Here's how the part is built. I have some questions about the finished solid (model axes, mm). A direction names the side the tool comes from. Round coordinates to 2 decimals unless told otherwise and drop trailing zeros. Loops run counter-clockwise (first coordinate to the right, second up) from the corner with the lowest first, then second, coordinate; pieces in that order, holes last. Notation, with made-up numbers: (56.25, 27) -> (110.25, 27) arc R31 ccw to (110.25, 55) -> close; hole circle Ø3 at (-34, 82.5). An arc over 180 degrees is marked (long way). Use one line per item in the form item = value. Start each with the question number.
Item 1: For faces 1 (the face through (42, 2, 68)), 2 (the face through (-93, 2, -10)), 3 (the face through (-80, 2, 1)), which set-ups out of +Z, -Z, +X, -X, +Y, -Y let a thin tool reach every point of the face, with its end or its side?
Item 2: I'm going to push flat-ended pins straight in: pin 1 Ø2.5 at (x, y) = (-44.5, 3) entering from +Z; pin 2 Ø2.5 at (x, y) = (72.5, 3) entering from +Z; pin 3 Ø1.9 at (x, z) = (-78, -48) entering from +Y; pin 4 Ø2.5 at (y, z) = (3, 36) entering from -X. Where does each tip first touch, or does it pass through?
Item 3: If we section it at B-B (z = 15): Write out the boundary of the cut face in (x, y).
Item 4: If I drill on L1, parallel to Z at x = -78, y = 2.4; L2, parallel to Z at x = 44.9, y = 4.05; L3, parallel to X at y = 4.6, z = -71.5, over which ranges is the centre line in solid material (lowest first)? Write a range as [from, to].
Item 5: Thinking about a two-plate mould opening in Z: for faces 4 (the face through (0, 2, 75)), 5 (the face through (100, 2, -48)), 6 (the face through (68, 2, -68)), which applies, released by +Z, released by -Z, zero draft, split by the parting line, or undercut?
Item 6: If we section it at A-A (x = 71): Write out the boundary of the cut face in (y, z), then the cut area to 3 significant figures.
Item 7: If we section it at C-C (y = 3.7): State how many separate pieces and enclosed holes the cut face has, then the cut area to 3 significant figures.
```python
from build123d import *

# Parameters (mm, degrees)
SKETCH1_R           = 1.55
SKETCH1_W           = 20
SKETCH1_H           = 15
SKETCH1_W_2         = 5
SKETCH1_H_2         = 25
BOSS_EXTRUDE2_DEPTH = 5


with BuildPart() as part:
    # Sketch1 → Boss-Extrude2 (new body)
    with BuildSketch(Plane(origin=(0, 0, 0), x_dir=(1, 0, 0), z_dir=(0, 1, 0))):
        Polygon((-25, -75), (25, -75), (25, -68), (60, -68), (60, -1), (100, -1), (100, 0), (100, 98), (-100, 98), (-100, 0), (-100, -1), (-60, -1), (-60, -68), (-25, -68), align=None)
        with Locations((-78, 48)):
            Circle(SKETCH1_R, mode=Mode.SUBTRACT)
        with Locations((78, 48)):
            Circle(SKETCH1_R, mode=Mode.SUBTRACT)
        with Locations((-40, 48)):
            Circle(SKETCH1_R, mode=Mode.SUBTRACT)
        with Locations((40, 48)):
            Circle(SKETCH1_R, mode=Mode.SUBTRACT)
        with Locations((-44.9, 26.9)):
            Circle(SKETCH1_R, mode=Mode.SUBTRACT)
        with Locations((44.9, 26.9)):
            Circle(SKETCH1_R, mode=Mode.SUBTRACT)
        with Locations((-44.9, -62.9)):
            Circle(SKETCH1_R, mode=Mode.SUBTRACT)
        with Locations((-44.9, -20.1)):
            Circle(SKETCH1_R, mode=Mode.SUBTRACT)
        with Locations((-54.9, -62.9)):
            Circle(SKETCH1_R, mode=Mode.SUBTRACT)
        with Locations((-54.9, -20.1)):
            Circle(SKETCH1_R, mode=Mode.SUBTRACT)
        with Locations((44.9, -62.9)):
            Circle(SKETCH1_R, mode=Mode.SUBTRACT)
        with Locations((54.9, -62.9)):
            Circle(SKETCH1_R, mode=Mode.SUBTRACT)
        with Locations((44.9, -20.1)):
            Circle(SKETCH1_R, mode=Mode.SUBTRACT)
        with Locations((54.9, -20.1)):
            Circle(SKETCH1_R, mode=Mode.SUBTRACT)
        with Locations((-55, 48)):
            Circle(SKETCH1_R, mode=Mode.SUBTRACT)
        with Locations((55, 48)):
            Circle(SKETCH1_R, mode=Mode.SUBTRACT)
        with Locations((-26.7, 10.2)):
            Circle(SKETCH1_R, mode=Mode.SUBTRACT)
        with Locations((26.7, 10.2)):
            Circle(SKETCH1_R, mode=Mode.SUBTRACT)
        with Locations((-40.5, 3.605469995)):
            Circle(SKETCH1_R, mode=Mode.SUBTRACT)
        with Locations((40.5, 3.605469995)):
            Circle(SKETCH1_R, mode=Mode.SUBTRACT)
        with Locations((-23, 53.5)):
            Circle(SKETCH1_R, mode=Mode.SUBTRACT)
        with Locations((23, 53.5)):
            Circle(SKETCH1_R, mode=Mode.SUBTRACT)
        with Locations((-55, 42)):
            Circle(SKETCH1_R, mode=Mode.SUBTRACT)
        with Locations((-55, 36)):
            Circle(SKETCH1_R, mode=Mode.SUBTRACT)
        with Locations((55, 36)):
            Circle(SKETCH1_R, mode=Mode.SUBTRACT)
        with Locations((55, 42)):
            Circle(SKETCH1_R, mode=Mode.SUBTRACT)
        with Locations((-78, 68.5)):
            Rectangle(SKETCH1_W, SKETCH1_H, mode=Mode.SUBTRACT)
        with Locations((78, 68.5)):
            Rectangle(SKETCH1_W, SKETCH1_H, mode=Mode.SUBTRACT)
        with Locations((-92.5, 22.5)):
            Rectangle(SKETCH1_W_2, SKETCH1_H_2, mode=Mode.SUBTRACT)
        with Locations((92.5, 22.5)):
            Rectangle(SKETCH1_W_2, SKETCH1_H_2, mode=Mode.SUBTRACT)
    extrude(amount=BOSS_EXTRUDE2_DEPTH)


solid = part.part
```
Values found:
q1.face_1 = +Z, +X, +Y, -Y
q1.face_2 = +Y, -Y
q1.face_3 = +Z, -X, +Y, -Y
q2.pin_1 = 68
q2.pin_2 = 1
q2.pin_3 = through
q2.pin_4 = -60
q3.outline = (-60, 0) -> (60, 0) -> (60, 5) -> (-60, 5) -> close
q4.L1 = [-98, -76], [-61, -49.55], [-46.45, 1]
q4.L2 = [-98, -28.45], [-25.35, 18.55], [21.65, 61.35], [64.45, 68]
q4.L3 = [-100, -88], [-68, 68], [88, 100]
q5.face_4 = released by +Z
q5.face_5 = zero draft
q5.face_6 = undercut
q6.outline = (0, -98) -> (5, -98) -> (5, -76) -> (0, -76) -> close; (0, -61) -> (5, -61) -> (5, 1) -> (0, 1) -> close
q6.area = 420 mm2
q7.separate_pieces = 1
q7.enclosed_holes = 30
q7.area = 27,100 mm2
